Here's how the part is built. I have some questions about the finished solid (model axes, mm). A direction names the side the tool comes from. Give positions to 0.01 mm unless a question says otherwise; leave off trailing zeros. Order: outer loops, then holes, each group sorted by start corner. A loop starts at its lowest first (then second) coordinate and runs counter-clockwise, first axis right, second up. Notation, with made-up numbers: (55.5, 23) - (90.5, 23) arc R21 cw to (90.5, 28) - close; hole circle Ø9 at (30, 43). An arc over 180 degrees is marked (long way). One line per question, with ' | ' between items.
from build123d import *

# Parameters (mm, degrees)
SKETCH_1_W      = 50.88
SKETCH_1_H      = 36.23
SKETCH_1_R      = 1.5
EXTRUDE_1_DEPTH = 3
SKETCH_2_W      = 6.361490509
SKETCH_2_H      = 8
SKETCH_2_R      = 2.5
SKETCH_2_W_2    = 6.95769393
EXTRUDE_2_DEPTH = 4


with BuildPart() as part:
    # 草图1 → 凸台-拉伸1 (new body)
    with BuildSketch(Plane.XY):
        with Locations((21.925, 0)):
            Rectangle(SKETCH_1_W, SKETCH_1_H)
        Circle(SKETCH_1_R, mode=Mode.SUBTRACT)
        with Locations((43.85, 0)):
            Circle(SKETCH_1_R, mode=Mode.SUBTRACT)
        with Locations((7.285, -5.115)):
            Circle(SKETCH_1_R, mode=Mode.SUBTRACT)
        with Locations((25.135, 9.235)):
            Circle(SKETCH_1_R, mode=Mode.SUBTRACT)
    extrude(amount=EXTRUDE_1_DEPTH)

    # 草图2 → 凸台-拉伸2 (add)
    # profile 1 of 2: a face of its own
    with BuildSketch(Plane(origin=(0, 0, 0), x_dir=(-1, 0, 0), z_dir=(0, 0, -1))):
        with Locations((0.334254746, 0)):
            Rectangle(SKETCH_2_W, SKETCH_2_H)
        Circle(SKETCH_2_R, mode=Mode.SUBTRACT)
    # profile 2 of 2: a face of its own
    with BuildSketch(Plane(origin=(0, 0, 0), x_dir=(-1, 0, 0), z_dir=(0, 0, -1))):
        with Locations((-43.886153035, 0)):
            Rectangle(SKETCH_2_W_2, SKETCH_2_H)
        with Locations((-43.85, 0)):
            Circle(SKETCH_2_R, mode=Mode.SUBTRACT)
    extrude(amount=EXTRUDE_2_DEPTH)


solid = part.part
1) Please list where these lines run through material, in increasing order: L1, parallel to Y at x = 0, z = 1.65 (3 decimals); L2, parallel to Y at x = 44, z = -2; L3, parallel to Z at x = 30, y = 5.5.
Model answer:
L1: y = -18.115 to -1.5, 1.5 to 18.115 | L2: y = -4 to -2.5, 2.5 to 4 | L3: z = 0 to 3
2) On a 3-axis mill with a long thin cutter (end or side, diameter ignored), from which of +Z, -Z, +X, -X, +Y, -Y can I reach the whole of each face in a straight line? I mean faces 1 (the face through (41.54, -0.96, -1.97)), 2 (the face through (0, 4, -2)), 3 (the face through (2.846, 0, -2)). Say none if no direction works.
Model answer:
face 1: -Z | face 2: -Z, +X, -X, +Y | face 3: -Z, +Y, -Y
3) I want a section at B-B (x = 0). List the corners of the cut face in (y, z) for me (3 decimals).
Model answer:
outline: (-18.115, 0) - (-4, 0) - (-4, -4) - (-2.5, -4) - (-2.5, 0) - (-1.5, 0) - (-1.5, 3) - (-18.115, 3) - close; (1.5, 0) - (2.5, 0) - (2.5, -4) - (4, -4) - (4, 0) - (18.115, 0) - (18.115, 3) - (1.5, 3) - close
4) I'm going to push flat-ended pins straight in: P1, Ø5.5, axis at x = 44, y = -1, coming from the -Z side; P2, Ø1.8, axis at x = 0, y = 0, coming from the +Z side; P3, Ø1.2, axis at x = 45, z = -2, coming from the +Y side; P4, Ø2, axis at x = 45.5, z = -2, coming from the -Y side. Where does each tip first touch, or does it pass through?
Model answer:
P1: stops at z = -4 | P2: passes through | P3: stops at y = 4 | P4: stops at y = -4
5) Thinking about a two-plate mould opening in Y: for faces 4 (the face through (22, 0, 3)), 5 (the face through (22, 18.115, 1)), 6 (the face through (44, -2, 0)), which applies, +Y half, -Y half, draft (parallel to the pull), parting line (faces both ways), or undercut?
Model answer:
face 4: draft | face 5: +Y half | face 6: undercut
6) I want a section at D-D (x = 30.5). List the corners of the cut face in (y, z) for me (3 decimals), plus the area to 3 significant figures.
Model answer:
outline: (-18.115, 0) - (18.115, 0) - (18.115, 3) - (-18.115, 3) - close | area: 109 mm2
7) I want a section at C-C (y = 8.5). List the corners of the cut face in (x, z) for me (3 decimals).
Model answer:
outline: (-3.515, 0) - (23.827, 0) - (23.827, 3) - (-3.515, 3) - close; (26.443, 0) - (47.365, 0) - (47.365, 3) - (26.443, 3) - close
8) I want a section at A-A (y = 0). State how many separate pieces and enclosed holes the cut face has, plus the area to 3 significant figures.
Model answer:
separate pieces: 3 | enclosed holes: 0 | area: 148 mm2
